Here's how the part is built. I have some questions about the finished solid (model axes, mm). A direction names the side the tool comes from. Round coordinates to 2 decimals unless told otherwise and drop trailing zeros. Write each loop counter-clockwise with the first axis right and the second up, starting at its lowest first coordinate (ties: lowest second). Pieces come first, ordered by that corner, then holes. Notation, with made-up numbers: (7, -2) -> (58, -2) arc R17 cw to (58, 16) -> close; hole circle Ø8 at (-13.75, 11.25). An arc over 180 degrees is marked (long way). Answer in a Markdown table with one row per item.
from build123d import *

# Parameters (mm, degrees)
ESQUISSE1_W             = 60.48
ESQUISSE1_H             = 36.81
BOSS_EXTRU_1_DEPTH      = 1.6
HOLES_R                 = 0.746107215
HOLES_R_2               = 0.75
HOLES_R_3               = 1.250449685
HOLES_R_4               = 0.749278137
ENL_V_MAT_EXTRU_1_DEPTH = 1.6
ESQUISSE4_R             = 0.375
ENL_V_MAT_EXTRU_2_DEPTH = 1.6
COMPOSANTS_W            = 10.427845653
COMPOSANTS_H            = 3.536930105
COMPOSANTS_W_2          = 3.243777278
COMPOSANTS_H_2          = 1.776354224
COMPOSANTS_W_3          = 2.973462505
COMPOSANTS_W_4          = 2.623427815
COMPOSANTS_H_3          = 1.178088166
COMPOSANTS_W_5          = 2.634336038
COMPOSANTS_H_4          = 1.145363495
BOSS_EXTRU_2_DEPTH      = 1.5
ESQUISSE6_W             = 19.651518654
ESQUISSE6_H             = 10.276618936
BOSS_EXTRU_3_DEPTH      = 10
ESQUISSE7_W             = 10
ESQUISSE7_H             = 10.276618936
ENL_V_MAT_EXTRU_3_DEPTH = 0.1


with BuildPart() as part:
    # Esquisse1 → Boss.-Extru.1 (new body)
    with BuildSketch(Plane.XY):
        Rectangle(ESQUISSE1_W, ESQUISSE1_H)
    extrude(amount=BOSS_EXTRU_1_DEPTH)

    # holes → Enlèv. mat.-Extru.1 (cut)
    with BuildSketch(Plane(origin=(0, 0, 0), x_dir=(-1, 0, 0), z_dir=(0, 0, -1))):
        with Locations((-26.820081416, 15.971189451)):
            Circle(HOLES_R)
        with Locations((-24.280081416, 15.971189451)):
            Circle(HOLES_R)
        with Locations((-21.740081416, 15.971189451)):
            Circle(HOLES_R)
        with Locations((-19.200081416, 15.971189451)):
            Circle(HOLES_R)
        with Locations((-16.660081416, 15.971189451)):
            Circle(HOLES_R)
        with Locations((-0.111966665, 15.971189451)):
            Circle(HOLES_R_2)
        with Locations((2.428033335, 15.971189451)):
            Circle(HOLES_R_2)
        with Locations((4.968033335, 15.971189451)):
            Circle(HOLES_R_2)
        with Locations((-2.651966665, 15.971189451)):
            Circle(HOLES_R_2)
        with Locations((-5.191966665, 15.971189451)):
            Circle(HOLES_R_2)
        with Locations((-8.714200976, -5.38768812)):
            Circle(HOLES_R_3)
        with Locations((23.712324903, -16.38246564)):
            Circle(HOLES_R_2)
        with Locations((26.252324903, -16.38246564)):
            Circle(HOLES_R_2)
        with Locations((28.792324903, -16.38246564)):
            Circle(HOLES_R_2)
        with Locations((21.172324903, -16.38246564)):
            Circle(HOLES_R_2)
        with Locations((-16.219684892, -13.565590628)):
            Circle(HOLES_R_2)
        with Locations((-20.031169083, -13.565590628)):
            Circle(HOLES_R_2)
        with Locations((4.79677487, -14.121575923)):
            Circle(HOLES_R_2)
        with Locations((8.63305215, -14.121575923)):
            Circle(HOLES_R_4)
    extrude(amount=-ENL_V_MAT_EXTRU_1_DEPTH, mode=Mode.SUBTRACT)

    # Esquisse4 → Enlèv. mat.-Extru.2 (cut)
    with BuildSketch(Plane.XY.offset(1.6)):
        with Locations((28.522800068, 2.172855337)):
            Circle(ESQUISSE4_R)
        with Locations((28.522800068, 4.712855337)):
            Circle(ESQUISSE4_R)
        with Locations((28.522800068, 7.252855337)):
            Circle(ESQUISSE4_R)
        with Locations((28.522800068, 9.792855337)):
            Circle(ESQUISSE4_R)
    extrude(amount=-ENL_V_MAT_EXTRU_2_DEPTH, mode=Mode.SUBTRACT)

    # composants → Boss.-Extru.2 (add)
    with BuildSketch(Plane.XY.offset(1.6)):
        with Locations((3.505618489, 0.895242457)):
            Rectangle(COMPOSANTS_W, COMPOSANTS_H)
        with Locations((16.297230516, 3.949212585)):
            Rectangle(COMPOSANTS_W_2, COMPOSANTS_H_2)
        with Locations((12.252163018, 3.949212585)):
            Rectangle(COMPOSANTS_W_3, COMPOSANTS_H_2)
        with Locations((5.088820687, 3.970981166)):
            Rectangle(COMPOSANTS_W_4, COMPOSANTS_H_3)
        with Locations((1.532739741, 3.987343502)):
            Rectangle(COMPOSANTS_W_5, COMPOSANTS_H_4)
    extrude(amount=BOSS_EXTRU_2_DEPTH)

    # Esquisse6 → Boss.-Extru.3 (add)
    with BuildSketch(Plane.XY.offset(1.6)):
        with Locations((-20.414240673, 10.357703845)):
            Rectangle(ESQUISSE6_W, ESQUISSE6_H)
    extrude(amount=BOSS_EXTRU_3_DEPTH)

    # Esquisse7 → Enlèv. mat.-Extru.3 (cut)
    with BuildSketch(Plane.ZY.offset(30.24)):
        with Locations((6.6, 10.357703845)):
            Rectangle(ESQUISSE7_W, ESQUISSE7_H)
    extrude(amount=-ENL_V_MAT_EXTRU_3_DEPTH, mode=Mode.SUBTRACT)


solid = part.part
1) I want a section at C-C, the plane y = 0. List the corners of the cut face in (x, z) for me, and give its area (3 significant figures).
Response:
| item | result |
|---|---|
| outline | (-30.24, 0) -> (30.24, 0) -> (30.24, 1.6) -> (8.72, 1.6) -> (8.72, 3.1) -> (-1.71, 3.1) -> (-1.71, 1.6) -> (-30.24, 1.6) -> close |
| area | 112 mm^2 |
2) I want a section at D-D, the plane z = 9.5. List the corners of the cut face in (x, y) for me, and give its area (3 significant figures).
Response:
| item | result |
|---|---|
| outline | (-30.14, 5.22) -> (-10.59, 5.22) -> (-10.59, 15.5) -> (-30.14, 15.5) -> close |
| area | 201 mm^2 |
3) For pin 1 (3 mm diameter, centred on y = 11, z = 4.5, fed in from +X); pin 2 (0.5 mm diameter, centred on x = 12.5, y = 4.5, fed in from +Z); pin 3 (1.4 mm diameter, centred on x = -21.17, y = -16.38, fed in from -Z); pin 4 (0.6 mm diameter, centred on y = 3.5, z = 2.5, fed in from +X), each with a flat end and sliding along its axis, tell me the tip position at first contact or that it passes through.
Response:
| item | result |
|---|---|
| pin 1 | stops at x = -10.59 |
| pin 2 | stops at z = 3.1 |
| pin 3 | passes through |
| pin 4 | stops at x = 17.92 |
4) We'd pull the mould along Y, two halves only. Please class faces 1 (the face through (0.21, 16.715, 0.789)), 2 (the face through (12, 3.061, 2)), 3 (the face through (-30.24, 0, 1)): +Y half, -Y half, draft (parallel to the pull), parting line (faces both ways), or undercut.
Response:
| item | result |
|---|---|
| face 1 | undercut |
| face 2 | -Y half |
| face 3 | draft |
5) Which directions (+Z, -Z, +X, -X, +Y, -Y) give clear straight access to the entire face, cutting with the end or side of a thin tool? Please do faces 4 (the face through (16, 4.837, 2)), 5 (the face through (17.919, 4, 2)), 6 (the face through (5, 3.382, 2)).
Response:
| item | result |
|---|---|
| face 4 | +Z, +X, -X, +Y |
| face 5 | +Z, +X, +Y, -Y |
| face 6 | +Z, -X |
6) I want a section at B-B, the plane x = -19. List the corners of the cut face in (y, z) for me (3 decimals).
Response:
| item | result |
|---|---|
| outline | (-18.405, 0) -> (18.405, 0) -> (18.405, 1.6) -> (15.496, 1.6) -> (15.496, 11.6) -> (5.219, 11.6) -> (5.219, 1.6) -> (-18.405, 1.6) -> close |
7) I need wall thicknesses on line 1 (X direction, y = 10, z = 6.5); line 2 (Y direction, x = -12, z = 2.25); line 3 (Z direction, x = 2, y = 15). Which ranges of each line are inside material? Lowest first, please. Write a range as [from, to].
Response:
| item | result |
|---|---|
| line 1 | x = [-30.14, -10.59] |
| line 2 | y = [5.22, 15.5] |
| line 3 | z = [0, 1.6] |
8) I want a section at A-A, the plane z = 2.25. List the corners of the cut face in (x, y) for me, and give its area (3 significant figures).
Response:
| item | result |
|---|---|
| outline | (-30.14, 5.22) -> (-10.59, 5.22) -> (-10.59, 15.5) -> (-30.14, 15.5) -> close; (-1.71, -0.87) -> (8.72, -0.87) -> (8.72, 2.66) -> (-1.71, 2.66) -> close; (0.22, 3.41) -> (2.85, 3.41) -> (2.85, 4.56) -> (0.22, 4.56) -> close; (3.78, 3.38) -> (6.4, 3.38) -> (6.4, 4.56) -> (3.78, 4.56) -> close; (10.77, 3.06) -> (13.74, 3.06) -> (13.74, 4.84) -> (10.77, 4.84) -> close; (14.68, 3.06) -> (17.92, 3.06) -> (17.92, 4.84) -> (14.68, 4.84) -> close |
| area | 255 mm^2 |
